```python
from build123d import *

# Parameters (mm, degrees)
F0_W     = 58
F0_H     = 20
F1_DEPTH = 4
F2_T     = -1
F3_W     = 1
F3_H     = 18
F4_DEPTH = 3
F5_R     = 0.5
F7_D     = 1
F7_DEPTH = 1


with BuildPart() as f1:
    # F0 (on Front) → F1 (new body)
    with BuildSketch(Plane.XZ):
        with Locations((9.587663, 9.659091)):
            Rectangle(F0_W, F0_H)
    extrude(amount=F1_DEPTH)

    # F2
    f2_openings = [f1.faces().sort_by_distance(p)[0] for p in [
        (9.587663, -4, 9.659091),
    ]]
    offset(amount=F2_T, openings=f2_openings)

    # F3 (on face) → F4 (cut)
    with BuildSketch(Plane.XZ.offset(4)):
        with Locations((-18.912337, 9.659091)):
            Rectangle(F3_W, F3_H)
        Polygon((38.587663, 0.659091), (37.587663, 0.659091), (-18.412337, 0.659091), (-19.412337, 0.659091), (-19.412337, -0.340909), (38.587663, -0.340909), align=None)
        with Locations((38.087663, 9.659091)):
            Rectangle(F3_W, F3_H)
    extrude(amount=-F4_DEPTH, mode=Mode.SUBTRACT)

    # F5
    f5_edges = [f1.edges().sort_by_distance(p)[0] for p in [
        (9.587663, 0, 19.659091),
    ]]
    fillet(f5_edges, radius=F5_R)

    # F7
    with Locations(Plane.XY.offset(19.659091)):
        with Locations((28.587663, -2.5)):
            Hole(F7_D / 2, depth=F7_DEPTH)


solid = f1.part
```
Geometry check sheet. Reference: the model listing, model coordinates, mm. A direction names the side the tool comes from. Give positions to 0.01 mm unless a question says otherwise; leave off trailing zeros. Write each loop counter-clockwise with the first axis right and the second up, starting at its lowest first coordinate (ties: lowest second). Pieces come first, ordered by that corner, then holes.
1) Release check for a two-part mould opening along X. For faces 1 (the flat face through (9, -2, 19.659)), 2 (the cylindrical face through (28.11, -2.35, 19.15)), 3 (the flat face through (-19.412, -0.7, 10.4)), 4 (the flat face through (38.588, -0.7, 10.4)) record: pulls with the +X half, pulls with the -X half, needs draft (parallel to the pull), parting line crosses it, or undercut.
2) Material ranges on L1, parallel to Z at x = 22, y = -2.1; L2, parallel to Y at x = -9, z = 3.75; L3, parallel to Z at x = 24.5, y = -0.25, recorded low to high.
3) Section check B-B, the plane x = 17. Record the boundary of the cut face in (y, z), and give its area (3 significant figures).
4) Gauge pin test, flat ends, axial feed: pin 1 (1.5 mm diameter, centred on x = 12, y = -3, fed in from -Z); pin 2 (1.5 mm diameter, centred on y = -2.5, z = 9.5, fed in from -X); pin 3 (9.5 mm diameter, centred on x = 14, z = 6.5, fed in from -Y). Record the tip position at first contact, or that the pin passes through.
5) Section check C-C, the plane z = 5. Record the boundary of the cut face in (x, y), and give its area (3 significant figures).
6) Access from +Z, -Z, +X, -X, +Y, -Y to the whole of each face (thin tool, end or side, straight path). Record for faces 5 (the flat face through (9, -1, 9)), 6 (the flat face through (9, -4, 19)).
7) Section check A-A, the plane y = -2.5. Record the boundary of the cut face in (x, z).
Computed:
1. face 1: needs draft
1. face 2: undercut
1. face 3: pulls with the -X half
1. face 4: pulls with the +X half
2. L1: z = 18.66 to 19.66
2. L2: y = -1 to 0
2. L3: z = -0.34 to 19.59
3. outline: (-4, 18.66) - (-1, 18.66) - (-1, -0.34) - (0, -0.34) - (0, 19.16) arc R0.5 ccw to (-0.5, 19.66) - (-4, 19.66) - close
3. area: 22.9 mm2
4. pin 1: stops at z = 18.66
4. pin 2: passes through
4. pin 3: stops at y = -1
5. outline: (-19.41, -1) - (38.59, -1) - (38.59, 0) - (-19.41, 0) - close
5. area: 58.0 mm2
6. face 5: -Z, +X, -X, -Y
6. face 6: +Z, -Z, +X, -X, -Y
7. outline: (-19.41, 18.66) - (28.09, 18.66) - (28.09, 19.66) - (-19.41, 19.66) - close; (29.09, 18.66) - (38.59, 18.66) - (38.59, 19.66) - (29.09, 19.66) - close
